```python
from build123d import *

# Parameters (mm, degrees)
SKETCH_1_R          = 8
EXTRUDE_1_DEPTH     = 40
CUT_EXTRUDE_START   = 20
SKETCH_2_W          = 30
SKETCH_2_H          = 45
CUT_EXTRUDE_1_DEPTH = 10
FILLET_1_R          = 3


with BuildPart() as part:
    # Эскиз1 → Бобышка-Вытянуть1 (new body)
    with BuildSketch(Plane.XY):
        with BuildLine():
            Line((0, 0), (30, 0))
            Line((30, 0), (30, 65))
            ThreePointArc((30, 65), (15, 80), (0, 65))
            Line((0, 65), (0, 0))
        make_face()
        with Locations((15, 65)):
            Circle(SKETCH_1_R, mode=Mode.SUBTRACT)
    extrude(amount=EXTRUDE_1_DEPTH)

    # Эскиз2 → Вырез-Вытянуть1 (cut, symmetric)
    with BuildSketch(Plane.XY.offset(CUT_EXTRUDE_START)):
        with Locations((15, 57.5)):
            Rectangle(SKETCH_2_W, SKETCH_2_H)
    extrude(amount=CUT_EXTRUDE_1_DEPTH, both=True, mode=Mode.SUBTRACT)

    # Скругление1
    fillet_1_edges = [part.edges().sort_by_distance(p)[0] for p in [
        (15, 35, 30),
        (15, 35, 10),
    ]]
    fillet(fillet_1_edges, radius=FILLET_1_R)


solid = part.part
```
The model under review builds one solid part; all positions refer to its coordinate system, in mm. A direction names the side the tool comes from. Round coordinates to 2 decimals unless told otherwise and drop trailing zeros. Loops run counter-clockwise (first coordinate to the right, second up) from the corner with the lowest first, then second, coordinate; pieces in that order, holes last.
Item 1: For faces 1 (the face through (15.21, 35.9, 29.14)), 2 (the face through (15, 80, 35)), list the 3-axis set-ups (+Z, -Z, +X, -X, +Y, -Y) from which the entire face can be reached by the end or side of a thin tool; tool diameter is ignored.
Determined:
face 1: +X, -X, +Y
face 2: +Z, -Z, +Y
Item 2: Mouldability with a two-part tool opening along Y and no side actions: class faces 3 (the face through (15, 80, 5)), 4 (the face through (13.959, 72.932, 34.93)), 5 (the face through (15, 41, 40)) as released by +Y, released by -Y, zero draft, split by the parting line, or undercut.
Determined:
face 3: released by +Y
face 4: undercut
face 5: zero draft
Item 3: Take a section at B-B (z = 35). Write out the cut boundary in (x, y), then the cut area to 3 significant figures.
Determined:
outline: (0, 0) - (30, 0) - (30, 65) arc R15 ccw to (0, 65) - close; hole circle Ø16 at (15, 65)
area: 2,100 mm2
Item 4: Take a section at D-D (x = 10.5). Write out the cut boundary in (y, z).
Determined:
outline: (0, 0) - (58.39, 0) - (58.39, 10) - (38, 10) arc R3 cw to (35, 13) - (35, 27) arc R3 cw to (38, 30) - (58.39, 30) - (58.39, 40) - (0, 40) - close; (71.61, 0) - (79.31, 0) - (79.31, 10) - (71.61, 10) - close; (71.61, 30) - (79.31, 30) - (79.31, 40) - (71.61, 40) - close
Item 5: Take a section at C-C (x = 24.75). Write out the cut boundary in (y, z), then the cut area to 3 significant figures.
Determined:
outline: (0, 0) - (76.4, 0) - (76.4, 10) - (38, 10) arc R3 cw to (35, 13) - (35, 27) arc R3 cw to (38, 30) - (76.4, 30) - (76.4, 40) - (0, 40) - close
area: 2,230 mm2
Item 6: Clearance check with flat-ended pins moving along their axes: pin 1 Ø2 at (x, z) = (13, 34) entering from +Y; pin 2 Ø4 at (x, z) = (13.5, 20) entering from +Y; pin 3 Ø14.5 at (x, y) = (15, 65) entering from +Z. State where each tip first meets the part, or that it passes through.
Determined:
pin 1: stops at y = 79.97
pin 2: stops at y = 35
pin 3: passes through
Item 7: Take a section at A-A (x = 15). Write out the cut boundary in (y, z).
Determined:
outline: (0, 0) - (57, 0) - (57, 10) - (38, 10) arc R3 cw to (35, 13) - (35, 27) arc R3 cw to (38, 30) - (57, 30) - (57, 40) - (0, 40) - close; (73, 0) - (80, 0) - (80, 10) - (73, 10) - close; (73, 30) - (80, 30) - (80, 40) - (73, 40) - close
Item 8: For line 1 (X direction, y = 65, z = 6.75); line 2 (Z direction, x = 23.5, y = 41.5); line 3 (Y direction, x = 15, z = 32.5), list the stretches that pass through material, from the lowest coordinate up.
Determined:
line 1: x = 0 to 7, 23 to 30
line 2: z = 0 to 10, 30 to 40
line 3: y = 0 to 57, 73 to 80
